Source: CAD feature listing. Evaluate the final solid. Frame: model axes, mm. Face numbers are marked on the shaded views. A direction names the side the tool comes from. Round coordinates to 2 decimals unless told otherwise and drop trailing zeros. Loops run counter-clockwise (first coordinate to the right, second up) from the corner with the lowest first, then second, coordinate; pieces in that order, holes last. Notation, with made-up numbers: (-9.75, 34) - (-5.75, 34) arc R26 cw to (-5.75, 52) - close; hole circle Ø9 at (80.25, -4). An arc over 180 degrees is marked (long way). Write item = value, one per line. Start each with the question number.
from build123d import *

# Parameters (mm, degrees)
F0_W     = 120
F0_H     = 120
F1_DEPTH = 60
F2_W     = 115
F2_H     = 115
F3_DEPTH = 59.8


# Not quite as in the source:
# - the program builds the solid bodies; features that only make, move or delete a surface that nothing else refers to are left out


with BuildPart() as f1:
    # F0 (on Front) → F1 (new body)
    with BuildSketch(Plane.XZ):
        Rectangle(F0_W, F0_H)
    extrude(amount=-F1_DEPTH)

    # F2 (on Front) → F3 (cut)
    with BuildSketch(Plane.XZ):
        Rectangle(F2_W, F2_H)
    extrude(amount=-F3_DEPTH, mode=Mode.SUBTRACT)


solid = f1.part
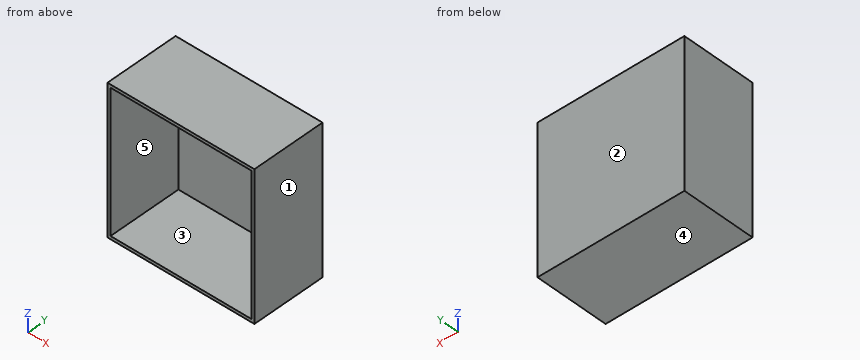
(1) Access query for the marked faces 4 and 5. Directions: +Z, -Z, +X, -X, +Y, -Y. A direction counts if a zero-diameter tool reaches every point of the face in a straight line with its end or side. Return the directions, or none.
(2) Cut plane C-C (x = -28). Output: boundary loops of the cut face in (y, z), and give its area (3 significant figures).
(3) Material intervals for line 1 along Z through (x, y) = (-19, 16.5); line 2 along Y through (x, z) = (-37.5, -46.5), sorted ascending. Write a range as from..to.
(4) Cut plane B-B (z = -22). Output: boundary loops of the cut face in (x, y), and give its area (3 significant figures).
(5) Mould query, pull axis X, two halves, no side actions, for the marked faces 1, 2 and 3. Classes: +X half, -X half, draft (parallel to the pull), parting line (faces both ways), or undercut.
(6) Pin query (flat end, axial travel): P1, Ø6, axis at x = 21.5, z = 10.5, coming from the -Y side. Return the tip coordinate at first contact, or that it passes through.
(7) Cut plane A-A (y = 6.5). Output: boundary loops of the cut face in (x, z), and give its area (4 significant figures).
Solution:
q1.face_4 = -Z, +X, -X, +Y, -Y
q1.face_5 = -Y
q2.outline = (0, -60) - (60, -60) - (60, 60) - (0, 60) - (0, 57.5) - (59.8, 57.5) - (59.8, -57.5) - (0, -57.5) - close
q2.area = 323 mm^2
q3.line_1 = -60..-57.5, 57.5..60
q3.line_2 = 59.8..60
q4.outline = (-60, 0) - (-57.5, 0) - (-57.5, 59.8) - (57.5, 59.8) - (57.5, 0) - (60, 0) - (60, 60) - (-60, 60) - close
q4.area = 323 mm^2
q5.face_1 = +X half
q5.face_2 = draft
q5.face_3 = undercut
q6.P1 = 59.8
q7.outline = (-60, -60) - (60, -60) - (60, 60) - (-60, 60) - close; hole (-57.5, -57.5) - (57.5, -57.5) - (57.5, 57.5) - (-57.5, 57.5) - close
q7.area = 1,175 mm^2
